Work out the finished part from the listing and answer in its coordinate system (mm). A direction names the side the tool comes from. Round coordinates to 2 decimals unless told otherwise and drop trailing zeros. Loops run counter-clockwise (first coordinate to the right, second up) from the corner with the lowest first, then second, coordinate; pieces in that order, holes last. Notation, with made-up numbers: (-21, 55) - (3, 55) arc R23 cw to (3, 71) - close; hole circle Ø7 at (62, 79.5). An arc over 180 degrees is marked (long way). Return JSON: item names as keys, results as strings.
from build123d import *

# Parameters (mm, degrees)
BOSS_EXTRUDE1_DEPTH          = 9
SKETCH2_R                    = 4
BOSS_EXTRUDE2_DEPTH          = 6.5
BOSS_EXTRUDE4_START          = 6.5
SKETCH4_R                    = 4
BOSS_EXTRUDE4_DEPTH          = 6.5
F_5_0_5_DIAMETER_HOLE1_D     = 5
F_5_0_5_DIAMETER_HOLE1_DEPTH = 23


# Read off the part's stored shape, not the designer's step: Boss-Extrude3, Boss-Extrude5
with BuildPart() as part:
    # Sketch1 → Boss-Extrude1 (new body)
    with BuildSketch(Plane(origin=(0, 4.5, 0), x_dir=(1, 0, 0), z_dir=(0, 1, 0))):
        with BuildLine():
            Line((-30, -82.5), (110, -82.5))
            ThreePointArc((110, -82.5), (114.5, -78), (110, -73.5))
            Line((110, -73.5), (-30, -73.5))
            ThreePointArc((-30, -73.5), (-34.5, -78), (-30, -82.5))
        make_face()
    extrude(amount=-BOSS_EXTRUDE1_DEPTH)

    # Sketch2 → Boss-Extrude2 (add)
    with BuildSketch(Plane(origin=(0, 4.5, 0), x_dir=(-1, 0, 0), z_dir=(0, 1, 0))):
        with Locations(Location((-40, 78, 0), (0, 0, 270))):
            Circle(SKETCH2_R)
    extrude(amount=BOSS_EXTRUDE2_DEPTH)

    # Boss-Extrude3 outline → Boss-Extrude3 (revolve)
    with BuildSketch(Plane(origin=(40, 0, 78), x_dir=(1, 0, 0), z_dir=(0, 0, 1))):
        with BuildLine():
            Line((2, 11), (2, 16.499999998))
            ThreePointArc((2, 16.499999998), (1.414213563, 17.914213562), (0, 18.5))
            Line((0, 18.5), (0, 11))
            Line((0, 11), (2, 11))
        make_face()
    revolve(axis=Axis((40, 0, 78), (0, 1, 0)))

    # Sketch4 → Boss-Extrude4 (add)
    with BuildSketch(Plane.XZ.offset(4.5).offset(BOSS_EXTRUDE4_START)):
        with Locations(Location((40, 78, 0), (0, 0, 270))):
            Circle(SKETCH4_R)
    extrude(amount=-BOSS_EXTRUDE4_DEPTH)

    # Boss-Extrude5 outline → Boss-Extrude5 (revolve)
    with BuildSketch(Plane(origin=(40, 0, 78), x_dir=(1, 0, 0), z_dir=(0, 0, 1))):
        with BuildLine():
            ThreePointArc((0, -18.5), (1.414213563, -17.914213562), (2, -16.499999998))
            Line((2, -16.499999998), (2, -11))
            Line((2, -11), (0, -11))
            Line((0, -11), (0, -18.5))
        make_face()
    revolve(axis=Axis((40, 0, 78), (0, 1, 0)))

    # Ø5.0 (5) Diameter Hole1
    with Locations(Plane(origin=(0, 4.5, 0), x_dir=(1, 0, 0), z_dir=(0, 1, 0))):
        with Locations((-30, -78), (110, -78)):
            Hole(F_5_0_5_DIAMETER_HOLE1_D / 2, depth=F_5_0_5_DIAMETER_HOLE1_DEPTH)


solid = part.part
1) Section D-D (y = 9) is taken. Give the vertices of the cut face in (x, z), and give its area (3 significant figures).
Verdict:
{"outline": "circle Ø8 at (40, 78)", "area": "50.3 mm2"}
2) Flat-ended cylindrical pins translate along their axes: pin 1 (4 mm diameter, centred on y = -9.5, z = 80, fed in from +X); pin 2 (4 mm diameter, centred on x = 64.5, z = 78, fed in from +Y); pin 3 (4.5 mm diameter, centred on x = 9, z = 76, fed in from -Y); pin 4 (3 mm diameter, centred on y = -1, z = 79.5, fed in from -X). Find the tip coordinate at first contact, or state that the pin passes through.
Verdict:
{"pin 1": "stops at x = 44", "pin 2": "stops at y = 4.5", "pin 3": "stops at y = -4.5", "pin 4": "stops at x = -34.5"}
3) Section B-B (y = 1) is taken. Give the vertices of the cut face in (x, z).
Verdict:
{"outline": "(-30, 73.5) - (110, 73.5) arc R4.5 ccw to (110, 82.5) - (-30, 82.5) arc R4.5 ccw to start; hole circle Ø5 at (-30, 78); hole circle Ø5 at (110, 78)"}
4) A tool of negligible diameter and unlimited length cuts with its end or side. For faces 4 (the flat face through (38, 11, 77)), 5 (the cylindrical face through (42.7, -7.8, 80.95)), 6 (the cylindrical face through (-34.5, 0.1, 77.9)), from which of +Z, -Z, +X, -X, +Y, -Y can it reach the whole face along a straight path? Write none if from no direction.
Verdict:
{"face 4": "+Y", "face 5": "-Y", "face 6": "-X, +Y, -Y"}
5) Section C-C (x = 64.5) is taken. Give the vertices of the cut face in (y, z).
Verdict:
{"outline": "(-4.5, 73.5) - (4.5, 73.5) - (4.5, 82.5) - (-4.5, 82.5) - close"}
6) Find the intervals of material crossed by L1, parallel to X at y = -0.5, z = 78; L2, parallel to Z at x = 110, y = -2; L3, parallel to Y at x = 19, z = 79.25, in increasing order.
Verdict:
{"L1": "x = -34.5 to -32.5, -27.5 to 107.5, 112.5 to 114.5", "L2": "z = 73.5 to 75.5, 80.5 to 82.5", "L3": "y = -4.5 to 4.5"}
7) Determine the mould class of faces 1 (the flat face through (42, -11, 77)), 2 (the cylindrical face through (40, -14, 76)), 3 (the cylindrical face through (-29.46, -0.06, 80.44)) for opening direction Z: pulls with the +Z half, pulls with the -Z half, needs draft (parallel to the pull), parting line crosses it, or undercut.
Verdict:
{"face 1": "needs draft", "face 2": "parting line crosses it", "face 3": "undercut"}
8) Section A-A (z = 78) is taken. Give the vertices of the cut face in (x, y).
Verdict:
{"outline": "(-34.5, -4.5) - (-32.5, -4.5) - (-32.5, 4.5) - (-34.5, 4.5) - close; (-27.5, -4.5) - (36, -4.5) - (36, -11) - (38, -11) - (38, -16.5) arc R2 ccw to (42, -16.5) - (42, -11) - (44, -11) - (44, -4.5) - (107.5, -4.5) - (107.5, 4.5) - (44, 4.5) - (44, 11) - (42, 11) - (42, 16.5) arc R2 ccw to (38, 16.5) - (38, 11) - (36, 11) - (36, 4.5) - (-27.5, 4.5) - close; (112.5, -4.5) - (114.5, -4.5) - (114.5, 4.5) - (112.5, 4.5) - close"}
